Here's how the part is built. I have some questions about the finished solid (model axes, mm). A direction names the side the tool comes from. Coordinates: 2 decimals unless noted, no trailing zeros. Write each loop counter-clockwise with the first axis right and the second up, starting at its lowest first coordinate (ties: lowest second). Pieces come first, ordered by that corner, then holes. Notation, with made-up numbers: M 48.25,37.25 L 77.25,37.25 A4 cw 77.25,42.25 Z; hole C 83,11 d3. An arc over 180 degrees is marked long. Use one line per item in the form item = value. Start each with the question number.
1. I want a section at A-A, the plane y = -3.5. List the corners of the cut face in (x, z) for me, plus the area to 3 significant figures.
2. On a 3-axis mill with a long thin cutter (end or side, diameter ignored), from which of +Z, -Z, +X, -X, +Y, -Y can I reach the whole of each face in a straight line? I mean faces 1 (the face through (51, -9, -20.274)), 2 (the face through (51, 12, -82.274)), 3 (the face through (50.068, 2, -46)). Say none if no direction works.
3. I want a section at C-C, the plane x = 46. List the corners of the cut face in (y, z) for me.
4. I want a section at B-B, the plane z = -72. List the corners of the cut face in (x, y) for me, plus the area to 3 significant figures.
5. I'm going to push flat-ended pins straight in: pin 1 Ø5 at (x, y) = (15.5, -1) entering from +Z; pin 2 Ø1 at (x, z) = (51, -64) entering from -Y; pin 3 Ø2 at (x, y) = (5, 2) entering from -Z. Where does each tip first touch, or does it pass through?
6. Thinking about a two-plate mould opening in Z: for faces 4 (the face through (25.732, 1.434, -17.275)), 5 (the face through (51, 1, -16.273)), 6 (the face through (51, -18.5, -18)), which applies, released by +Z, released by -Z, zero draft, split by the parting line, or undercut?
7. I want a section at D-D, the plane x = -30. List the corners of the cut face in (y, z) for me, plus the area to 3 significant figures.
8. Please list where this line runs through material, in increasing order: line 1 along Y through (x, z) = (-3.5, -19.5). Write a range as [from, to].
Autodesk Inventor part; units mm, degrees
ref_plane "YZ Plane" through (0, 0, 0) normal (1, 0, 0) x (0, 1, 0)
ref_plane "XZ Plane" through (0, 0, 0) normal (0, 1, 0) x (-1, 0, 0)
ref_plane "XY Plane" through (0, 0, 0) normal (0, 0, 1) x (1, 0, 0)
sketch "Skizze1" plane through (0, 0, 0) normal (0, 1, 0) x (-1, 0, 0)
  line L0 (37.9316, -16.2735) -> (-2.0684, -16.2735)
  line L1 (-2.0684, -16.2735) -> (-2.0684, -86.2735)
  line L2 (-2.0684, -86.2735) -> (37.9316, -86.2735)
  line L3 (37.9316, -86.2735) -> (37.9316, -16.2735)
  point P0 (0, 0)
  dimension "d0" = 70
  dimension "d1" = 40
extrude "Extrusion1" add sketch "Skizze1" along normal blind 3
fillet "Rundung1" radius 1 4 edges at (-37.9316, 1.5, -16.2735) (-37.9316, 1.5, -86.2735) (2.0684, 1.5, -86.2735) (2.0684, 1.5, -16.2735)
sketch "Skizze2" plane through (2.0684, 0, -17.2735) normal (1, 0, 0) x (0, 0, -1)
  circle A0 centre (1.5, 1.5) radius 1.5
  circle A1 centre (66.5, 1.5) radius 1.5
  line L0 (0, 3) -> (68, 3)
  line L1 (0, 0) -> (0, 3)
  line L2 (68, 3) -> (68, 0)
  point P0 (-17.2735, 0)
  dimension "d5" = 3
  dimension "d6" = 3
  dimension "d7" = 1.5
  dimension "d8" = 1.5
  dimension "d9" = 1.5
  dimension "d10" = 1.5
extrude "Extrusion2" add sketch "Skizze2" along normal blind 50 contours A0 | A1
sketch "Skizze3" plane through (52.0684, 1.5, -18.7735) normal (1, 0, 0) x (0, 0, -1)
  line L0 (-2.5, 1.5) -> (67.5, 1.5)
  line L1 (67.5, 1.5) -> (67.5, -1.5)
  line L2 (67.5, -1.5) -> (-2.5, -1.5)
  line L3 (-2.5, -1.5) -> (-2.5, 1.5)
  circle A0 centre (0, 0) radius 1.5
  circle A1 centre (65, 0) radius 1.5
  line L4 (-2.5, 20) -> (1.5, 20)
  line L5 (1.5, 20) -> (1.5, -20)
  line L6 (1.5, -20) -> (-2.5, -20)
  line L7 (-2.5, -20) -> (-2.5, 20)
  line L8 (67.5, 20) -> (63.5, 20)
  line L9 (63.5, 20) -> (63.5, -20)
  line L10 (63.5, -20) -> (67.5, -20)
  line L11 (67.5, -20) -> (67.5, 20)
  point P0 (-18.7735, -1.5)
  dimension "d13" = 1.5
  dimension "d14" = 1.5
  dimension "d16" = 2.5
  dimension "d17" = 2.5
  dimension "d20" = 40
  dimension "d21" = 20
extrude "Extrusion4" add sketch "Skizze3" against normal blind 2
properties part number "Spielstraßenschild_gesamt"
Answer list:
q1.outline = M 50.07,-86.27 L 52.07,-86.27 L 52.07,-82.27 L 50.07,-82.27 Z; M 50.07,-20.27 L 52.07,-20.27 L 52.07,-16.27 L 50.07,-16.27 Z
q1.area = 16.0 mm²
q2.face_1 = +X, -X, -Y
q2.face_2 = +X, -X, +Y
q2.face_3 = none
q3.outline = C 1.5,-83.77 d3; C 1.5,-18.77 d3
q4.outline = M -37.93,0 L 2.07,0 L 2.07,3 L -37.93,3 Z; M 50.07,0 L 52.07,0 L 52.07,3 L 50.07,3 Z
q4.area = 126 mm²
q5.pin_1 = -17.27
q5.pin_2 = 0
q5.pin_3 = -85.27
q6.face_4 = undercut
q6.face_5 = released by +Z
q6.face_6 = zero draft
q7.outline = M 0,-86.27 L 3,-86.27 L 3,-16.27 L 0,-16.27 Z
q7.area = 210 mm²
q8.line_1 = [0, 3]
